Here's how the part is built. I have some questions about the finished solid (model axes, mm). A direction names the side the tool comes from. Coordinates: 2 decimals unless noted, no trailing zeros. Write each loop counter-clockwise with the first axis right and the second up, starting at its lowest first coordinate (ties: lowest second). Pieces come first, ordered by that corner, then holes.
Item 1: I'm going to push flat-ended pins straight in: P1, Ø3, axis at x = -0.5, z = 13, coming from the -Y side; P2, Ø0.6, axis at x = -5, y = 1, coming from the -Z side. Where does each tip first touch, or does it pass through?
Item 2: I want a section at B-B (x = 4.5). Please give me the cut outline in (y, z), and give its area (3 significant figures).
Item 3: For faces 1 (the face through (-4, 1, 16)), 2 (the face through (-5, 1, -15.5)), 3 (the face through (5, 1, 15.5)), which set-ups out of +Z, -Z, +X, -X, +Y, -Y let a thin tool reach every point of the face, with its end or its side?
Item 4: I want a section at A-A (y = 0.75). Please give me the cut outline in (x, z), and give its area (3 significant figures).
Item 5: Please list where this line runs through material, in increasing order: line 1 (Z direction, x = 5, y = 0.4).
from build123d import *

# Parameters (mm, degrees)
SKETCH1_W           = 12
SKETCH1_H           = 31
BOSS_EXTRUDE1_DEPTH = 1.3
SKETCH2_W           = 8
SKETCH2_H           = 1.4
BOSS_EXTRUDE2_DEPTH = 1.3


with BuildPart() as part:
    # Sketch1 → Boss-Extrude1 (new body)
    with BuildSketch(Plane(origin=(0, 0, 0), x_dir=(1, 0, 0), z_dir=(0, 1, 0))):
        Rectangle(SKETCH1_W, SKETCH1_H)
    extrude(amount=BOSS_EXTRUDE1_DEPTH)

    # Sketch2 → Boss-Extrude2 (add)
    with BuildSketch(Plane(origin=(0, 1.3, 0), x_dir=(1, 0, 0), z_dir=(0, 1, 0))):
        with Locations((0, 16.2)):
            Rectangle(SKETCH2_W, SKETCH2_H)
        with Locations((0, -16.2)):
            Rectangle(SKETCH2_W, SKETCH2_H)
    extrude(amount=-BOSS_EXTRUDE2_DEPTH)


solid = part.part
Answer:
1. P1: stops at y = 0
1. P2: stops at z = -15.5
2. outline: (0, -15.5) - (1.3, -15.5) - (1.3, 15.5) - (0, 15.5) - close
2. area: 40.3 mm2
3. face 1: +Z, -X, +Y, -Y
3. face 2: -Z, -X, +Y, -Y
3. face 3: +Z, +X, +Y, -Y
4. outline: (-6, -15.5) - (-4, -15.5) - (-4, -16.9) - (4, -16.9) - (4, -15.5) - (6, -15.5) - (6, 15.5) - (4, 15.5) - (4, 16.9) - (-4, 16.9) - (-4, 15.5) - (-6, 15.5) - close
4. area: 394 mm2
5. line 1: z = -15.5 to 15.5
